Build history of the part. All positions in model axes, mm. A direction names the side the tool comes from. Coordinates: 2 decimals unless noted, no trailing zeros. Order: outer loops, then holes, each group sorted by start corner. A loop starts at its lowest first (then second) coordinate and runs counter-clockwise, first axis right, second up. Notation, with made-up numbers: (10.5, 77) - (62.5, 77) arc R28 cw to (62.5, 102) - close; hole circle Ø7 at (-30, 17). An arc over 180 degrees is marked (long way). Write each question's results on one line, items separated by ' | '.
from build123d import *

# Parameters (mm, degrees)
BOSS_EXTRUDE1_DEPTH = 381
SHELL1_T            = -4.7625
SKETCH3_W           = 63.5
SKETCH3_H           = 4.7625
BOSS_EXTRUDE2_DEPTH = 381


with BuildPart() as part:
    # Sketch1 → Boss-Extrude1 (new body)
    with BuildSketch(Plane.XY):
        with BuildLine():
            Line((-50.652428891, 63.5), (50.652428891, 63.5))
            ThreePointArc((50.652428891, 63.5), (59.737033544, 59.737033544), (63.5, 50.652428891))
            Line((63.5, 50.652428891), (63.5, -50.652428891))
            ThreePointArc((63.5, -50.652428891), (59.737033544, -59.737033544), (50.652428891, -63.5))
            Line((50.652428891, -63.5), (-50.652428891, -63.5))
            ThreePointArc((-50.652428891, -63.5), (-59.737033544, -59.737033544), (-63.5, -50.652428891))
            Line((-63.5, -50.652428891), (-63.5, 50.652428891))
            ThreePointArc((-63.5, 50.652428891), (-59.737033544, 59.737033544), (-50.652428891, 63.5))
        make_face()
    extrude(amount=-BOSS_EXTRUDE1_DEPTH)

    # Shell1
    shell1_openings = [part.faces().sort_by_distance(p)[0] for p in [
        (0, 0, -381),
        (0, 0, 0),
    ]]
    offset(amount=SHELL1_T, openings=shell1_openings, kind=Kind.INTERSECTION)

    # Sketch3 → Boss-Extrude2 (add)
    with BuildSketch(Plane.XY):
        with Locations((0, -56.35625)):
            Rectangle(SKETCH3_W, SKETCH3_H)
    extrude(amount=-BOSS_EXTRUDE2_DEPTH)


solid = part.part
1. Band-saw the part on B-B on x = -20.5. Give the cut face in (y, z) (1 decimal).
Solved:
outline: (-63.5, -381) - (-54, -381) - (-54, 0) - (-63.5, 0) - close; (58.7, -381) - (63.5, -381) - (63.5, 0) - (58.7, 0) - close
2. Probe line 1 (Y direction, x = -5, z = -129.5) (1 decimal); line 2 (X direction, y = 33, z = -314). List the from-to ranges inside material, lowest first.
Solved:
line 1: y = -63.5 to -54, 58.7 to 63.5 | line 2: x = -63.5 to -58.74, 58.74 to 63.5
3. Band-saw the part on A-A on y = -30. Give the cut face in (x, z).
Solved:
outline: (-63.5, -381) - (-58.74, -381) - (-58.74, 0) - (-63.5, 0) - close; (58.74, -381) - (63.5, -381) - (63.5, 0) - (58.74, 0) - close
4. Tool access for faces 5 (the face through (-59.637, -59.836, -187.833)), 6 (the face through (56.43, -56.31, -187.83)): list every direction of +Z, -Z, +X, -X, +Y, -Y with a clear straight run to the whole face (end or side of a thin tool).
Solved:
face 5: +Z, -Z, -X, -Y | face 6: +Z, -Z
5. Drop flat-ended pins along their axis: pin 1 Ø5 at (y, z) = (-57.5, -177.5) entering from +X; pin 2 Ø5 at (y, z) = (-56.5, -269) entering from -X. Give the stop position or say it passes through.
Solved:
pin 1: stops at x = 62.74 | pin 2: stops at x = -63.06
6. Two-plate mould, pull along X, no slides. Class faces 1 (the face through (41, -58.738, -188)), 2 (the face through (-63.5, -1, -188)), 3 (the face through (56.31, 56.43, -187.83)), 4 (the face through (63.5, 1, -188)): +X half, -X half, draft (parallel to the pull), parting line (faces both ways), or undercut.
Solved:
face 1: undercut | face 2: -X half | face 3: undercut | face 4: +X half
